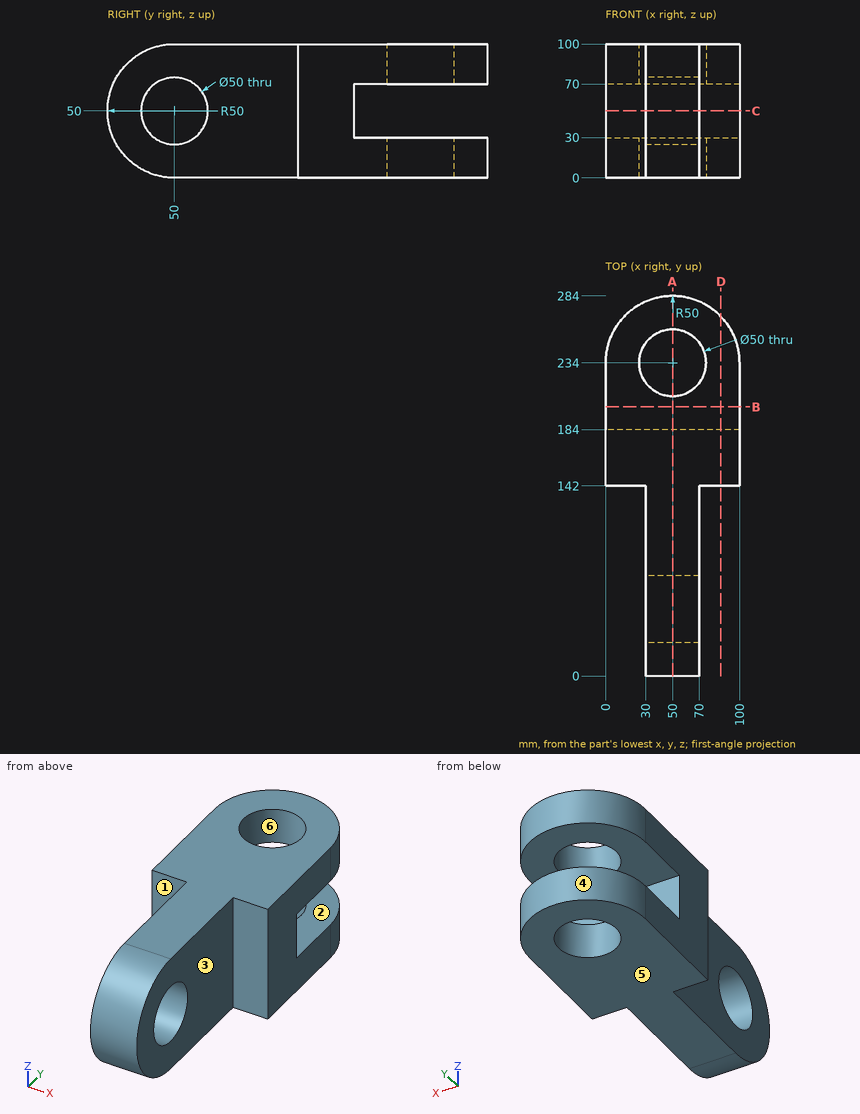
The figure shows three views and two pictorial views of one solid part (mm, origin at its lowest corner). Answer the questions. A direction names the side the tool comes from. Coordinates: 2 decimals unless noted, no trailing zeros. Loops run counter-clockwise (first coordinate to the right, second up) from the corner with the lowest first, then second, coordinate; pieces in that order, holes last. Notation, with made-up numbers: (-16.75, 16.5) -> (25.25, 16.5) arc R26 cw to (25.25, 30.5) -> close; hole circle Ø2 at (3.25, 75.5). An arc over 180 degrees is marked (long way). Use one line per item in the form item = value. Start each with the question number.
Item 1: A tool of negligible diameter and unlimited length cuts with its end or side. For the marked faces 1, 2 and 3, from which of +Z, -Z, +X, -X, +Y, -Y can it reach the whole face along a straight path? Write none if from no direction.
Item 2: The part is cut by section A-A on x = 50. Determine the outline of the cut face in (y, z).
Item 3: Consider L1, parallel to Y at x = 51, z = 50; L2, parallel to Y at x = 16, z = 60.5; L3, parallel to Y at x = 34.5, z = 92. Determine where each line is inside the solid, lowest interval first. Write a range as [from, to].
Item 4: The part is cut by section B-B on y = 201. Determine the outline of the cut face in (x, z), then the cut area to 3 significant figures.
Item 5: The part is cut by section D-D on x = 86. Determine the outline of the cut face in (y, z).
Item 6: The part is cut by section C-C on z = 50. Determine the outline of the cut face in (x, y), then the cut area to 3 significant figures.
Item 7: The mould has two halves that part along X. Classify the marked faces 4, 5 and 6: released by +X, released by -X, zero draft, split by the parting line, or undercut.
Item 8: Flat-ended cylindrical pins translate along their axes: pin 1 Ø1.5 at (y, z) = (96, 86) entering from -X; pin 2 Ø1.5 at (x, z) = (56.5, 25) entering from +Y; pin 3 Ø9 at (x, z) = (9, 74.5) entering from -Y. Find the tip coordinate at first contact, or state that the pin passes through.
Answer key:
q1.face_1 = +Z, -Z, -X, -Y
q1.face_2 = +X, -X, +Y
q1.face_3 = +Z, -Z, +X, -Y
q2.outline = (50, 0) -> (209, 0) -> (209, 30) -> (184, 30) -> (184, 70) -> (209, 70) -> (209, 100) -> (50, 100) arc R50 ccw to start; (259, 0) -> (284, 0) -> (284, 30) -> (259, 30) -> close; (259, 70) -> (284, 70) -> (284, 100) -> (259, 100) -> close; hole circle Ø50 at (50, 50)
q3.L1 = [0, 25], [75, 184]
q3.L2 = [142, 184]
q3.L3 = [22.87, 214.38], [253.62, 281.54]
q4.outline = (0, 0) -> (100, 0) -> (100, 30) -> (0, 30) -> close; (0, 70) -> (100, 70) -> (100, 100) -> (0, 100) -> close
q4.area = 6,000 mm2
q5.outline = (142, 0) -> (268.7, 0) -> (268.7, 30) -> (184, 30) -> (184, 70) -> (268.7, 70) -> (268.7, 100) -> (142, 100) -> close
q6.outline = (0, 142) -> (30, 142) -> (30, 75) -> (70, 75) -> (70, 142) -> (100, 142) -> (100, 184) -> (0, 184) -> close; (30, 0) -> (70, 0) -> (70, 25) -> (30, 25) -> close
q6.area = 7,880 mm2
q7.face_4 = split by the parting line
q7.face_5 = zero draft
q7.face_6 = undercut
q8.pin_1 = 30
q8.pin_2 = 283.67
q8.pin_3 = 142
